Build history of the part. All positions in model axes, mm. A direction names the side the tool comes from. Give positions to 0.01 mm unless a question says otherwise; leave off trailing zeros. Order: outer loops, then holes, each group sorted by start corner. A loop starts at its lowest first (then second) coordinate and runs counter-clockwise, first axis right, second up. Notation, with made-up numbers: M 49.5,3.5 L 93.5,3.5 A31 cw 93.5,40.5 Z; hole C -19,59.25 d1. An arc over 180 degrees is marked long. One line per item, written item: value.
from build123d import *

# Parameters (mm, degrees)
CROQUIS1_R              = 2.4
SALIENTE_EXTRUIR1_DEPTH = 3
SALIENTE_EXTRUIR2_DEPTH = 6


with BuildPart() as part:
    # Croquis1 → Saliente-Extruir1 (new body)
    with BuildSketch(Plane(origin=(0, 0, 0), x_dir=(1, 0, 0), z_dir=(0, 1, 0))):
        with BuildLine():
            Line((35.117506554, -10.768616799), (17.851894103, -10.768616799))
            Line((17.851894103, -10.768616799), (17.851894103, -15.511473942))
            ThreePointArc((17.851894103, -15.511473942), (16.931372558, -17.73380954), (14.70903696, -18.654331085))
            Line((14.70903696, -18.654331085), (11.280465531, -18.654331085))
            ThreePointArc((11.280465531, -18.654331085), (9.058129933, -17.73380954), (8.137608389, -15.511473942))
            Line((8.137608389, -15.511473942), (8.137608389, 1.036415275))
            ThreePointArc((8.137608389, 1.036415275), (9.058129933, 3.258750873), (11.280465531, 4.179272418))
            Line((11.280465531, 4.179272418), (14.70903696, 4.179272418))
            ThreePointArc((14.70903696, 4.179272418), (16.931372558, 3.258750873), (17.851894103, 1.036415275))
            Line((17.851894103, 1.036415275), (17.851894103, -3.797188228))
            Line((17.851894103, -3.797188228), (35.117506554, -3.797188228))
            ThreePointArc((35.117506554, -3.797188228), (42.791315147, -7.282902513), (35.117506554, -10.768616799))
        make_face()
        with Locations(Location((38.162743718, -7.282902513, 0), (0, 0, 270))):
            Circle(CROQUIS1_R, mode=Mode.SUBTRACT)
    extrude(amount=SALIENTE_EXTRUIR1_DEPTH)

    # Croquis2 → Saliente-Extruir2 (add)
    with BuildSketch(Plane(origin=(0, 3, 0), x_dir=(1, 0, 0), z_dir=(0, 1, 0))):
        with BuildLine():
            Line((13.22040734, -0.732902513), (13.22040734, -1.732902513))
            Line((13.22040734, -1.732902513), (17.851894103, -1.732902513))
            Line((17.851894103, -1.732902513), (17.851894103, 1.036415275))
            ThreePointArc((17.851894103, 1.036415275), (16.931372558, 3.258750873), (14.70903696, 4.179272418))
            Line((14.70903696, 4.179272418), (11.280465531, 4.179272418))
            ThreePointArc((11.280465531, 4.179272418), (9.058129933, 3.258750873), (8.137608389, 1.036415275))
            Line((8.137608389, 1.036415275), (8.137608389, -0.732902513))
            Line((8.137608389, -0.732902513), (13.22040734, -0.732902513))
        make_face()
        with BuildLine():
            Line((17.851894103, -12.832902513), (13.22040734, -12.832902513))
            Line((13.22040734, -12.832902513), (13.22040734, -13.832902513))
            Line((13.22040734, -13.832902513), (8.137608389, -13.832902513))
            Line((8.137608389, -13.832902513), (8.137608389, -15.511473942))
            ThreePointArc((8.137608389, -15.511473942), (9.058129933, -17.73380954), (11.280465531, -18.654331085))
            Line((11.280465531, -18.654331085), (14.70903696, -18.654331085))
            ThreePointArc((14.70903696, -18.654331085), (16.931372558, -17.73380954), (17.851894103, -15.511473942))
            Line((17.851894103, -15.511473942), (17.851894103, -12.832902513))
        make_face()
    extrude(amount=SALIENTE_EXTRUIR2_DEPTH)


solid = part.part
1) Mould opens along X. For faces 6 (the face through (11, 6, 0.733)), 7 (the face through (35.82, 1.48, 6.76)), 8 (the face through (16.96, 4.44, -3.23)), 9 (the face through (13.22, 6, 13)) say: released by +X, released by -X, zero draft, split by the parting line, or undercut.
Check values:
face 6: zero draft
face 7: undercut
face 8: released by +X
face 9: released by -X
2) Saw through at A-A, the plane z = 7.5. Write the cut outline in (x, y), then the cut area to 3 significant figures.
Check values:
outline: M 8.14,0 L 35.77,0 L 35.77,3 L 8.14,3 Z; M 40.55,0 L 42.79,0 L 42.79,3 L 40.55,3 Z
area: 89.6 mm^2
3) Saw through at D-D, the plane x = 36.5. Write the cut outline in (y, z), then the cut area to 3 significant figures.
Check values:
outline: M 0,2.96 L 3,2.96 L 3,5.55 L 0,5.55 Z; M 0,9.01 L 3,9.01 L 3,11.6 L 0,11.6 Z
area: 15.5 mm^2
4) Pin check, flat tips, straight feed: pin 1 (1.4 mm diameter, centred on x = 16, y = 7, fed in from -Z); pin 2 (2.5 mm diameter, centred on x = 22, y = 1.5, fed in from -Z); pin 3 (1.5 mm diameter, centred on y = 5, z = 12.5, fed in from -X). Stop position of each tip, or through.
Check values:
pin 1: z = -4.12
pin 2: z = 3.8
pin 3: x = 13.22
5) Saw through at B-B, the plane x = 12. Write the cut outline in (y, z), then the cut area to 3 significant figures.
Check values:
outline: M 0,-4.18 L 9,-4.18 L 9,0.73 L 3,0.73 L 3,13.83 L 9,13.83 L 9,18.65 L 0,18.65 Z
area: 127 mm^2
6) Saw through at C-C, the plane y = 1. Write the cut outline in (x, z), then the cut area to 3 significant figures.
Check values:
outline: M 8.14,-1.04 A3.14 ccw 11.28,-4.18 L 14.71,-4.18 A3.14 ccw 17.85,-1.04 L 17.85,3.8 L 35.12,3.8 A4.63 ccw long 35.12,10.77 L 17.85,10.77 L 17.85,15.51 A3.14 ccw 14.71,18.65 L 11.28,18.65 A3.14 ccw 8.14,15.51 Z; hole C 38.16,7.28 d4.8
area: 375 mm^2
7) Drill centre lines: probe 1 along Z at (x, y) = (11.5, 6); probe 2 along Z at (x, y) = (33, 2.5); probe 3 along X at (y, z) = (7.25, 0.5). Where is each one in solid material? Low to high. Write a range as from..to.
Check values:
probe 1: -4.18..0.73, 13.83..18.65
probe 2: 3.8..10.77
probe 3: 8.14..17.85
8) Tool access for faces 1 (the face through (13.22, 6, 1)), 2 (the face through (26, 1, 3.797)), 3 (the face through (27, 1, 10.769)), 4 (the face through (16, 6, 1.733)), 5 (the face through (13, 9, 16)): list every direction of +Z, -Z, +X, -X, +Y, -Y with a clear straight run to the whole face (end or side of a thin tool).
Check values:
face 1: -X, +Y
face 2: -Z, +Y, -Y
face 3: +Z, +Y, -Y
face 4: +X, -X, +Y
face 5: +Z, -Z, +X, -X, +Y
